The drawing under review shows one solid part. Ordinate dimensions are in mm from its lowest x, y, z. Give positions to 0.01 mm unless a question says otherwise; leave off trailing zeros. Order: outer loops, then holes, each group sorted by start corner. A loop starts at its lowest first (then second) coordinate and runs counter-clockwise, first axis right, second up. Notation, with made-up numbers: (10.5, -38) -> (31.5, -38) arc R29 cw to (31.5, 0) -> close; hole circle Ø1 at (32.5, -3.75). An arc over 180 degrees is marked (long way). Return JSON: item names as keys, results as strings. Group by question number.
1) Add section C-C (y = 0.6). Give the boundary of the cut face in (x, z), then the cut area to 3 significant figures.
2) Add section D-D (x = 48.5). Give the boundary of the cut face in (y, z), then the cut area to 3 significant figures.
3) To check wall thickness, follow line 1 along X through (y, z) = (1.95, 22.75); line 2 along Z through (x, y) = (4, 2); line 3 along X through (y, z) = (2.45, 41.5). State the ranges of each line that lie inside material, in increasing order.
4) Add section B-B (z = 20). Give the boundary of the cut face in (x, y).
5) Add section A-A (x = 4). Give the boundary of the cut face in (y, z).
6) Insertion check: P1, Ø2, axis at x = 4, z = 41.5, coming from the -Y side (3 decimals). The pin has a flat end and moves straight along its axis. Give the tip position at first contact, or say it passes through.
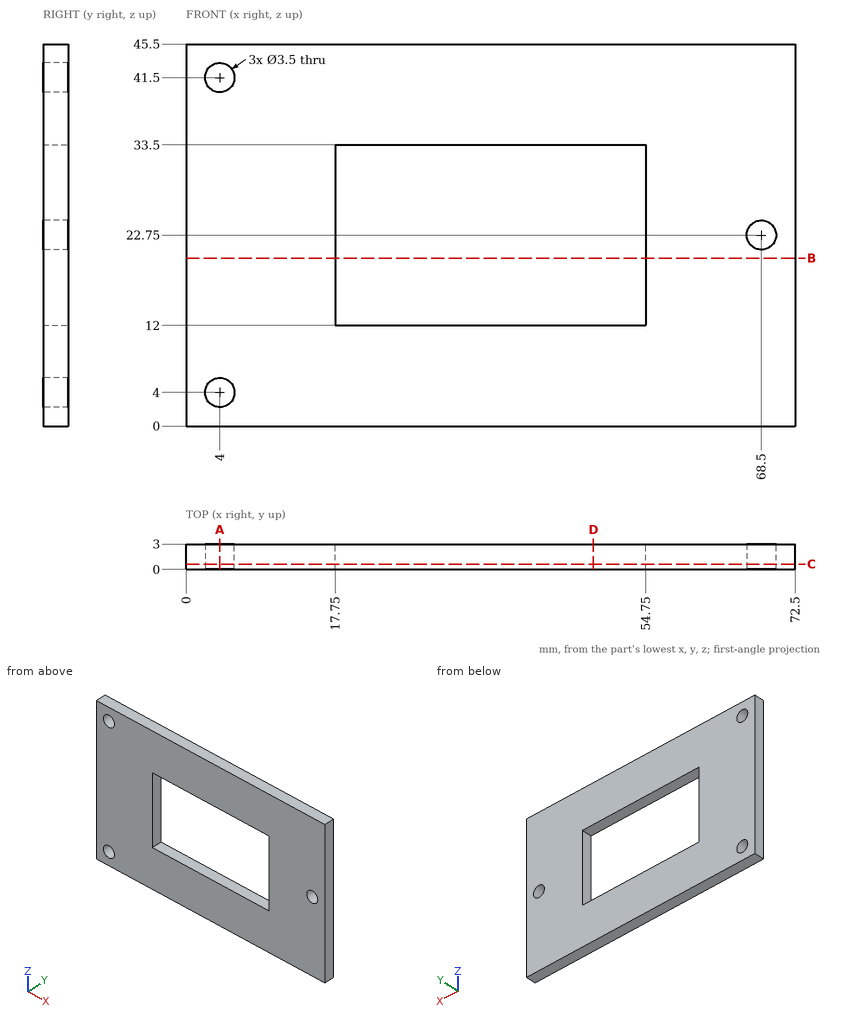
Evaluation:
{
 "1": {"outline": "(0, 0) -> (72.5, 0) -> (72.5, 45.5) -> (0, 45.5) -> close; hole circle Ø3.5 at (4, 4); hole circle Ø3.5 at (4, 41.5); hole (17.75, 12) -> (54.75, 12) -> (54.75, 33.5) -> (17.75, 33.5) -> close; hole circle Ø3.5 at (68.5, 22.75)", "area": "2,470 mm^2"},
 "2": {"outline": "(0, 0) -> (3, 0) -> (3, 12) -> (0, 12) -> close; (0, 33.5) -> (3, 33.5) -> (3, 45.5) -> (0, 45.5) -> close", "area": "72.0 mm^2"},
 "3": {"line 1": "0 to 17.75, 54.75 to 66.75, 70.25 to 72.5", "line 2": "0 to 2.25, 5.75 to 39.75, 43.25 to 45.5", "line 3": "0 to 2.25, 5.75 to 72.5"},
 "4": {"outline": "(0, 0) -> (17.75, 0) -> (17.75, 3) -> (0, 3) -> close; (54.75, 0) -> (72.5, 0) -> (72.5, 3) -> (54.75, 3) -> close"},
 "5": {"outline": "(0, 0) -> (3, 0) -> (3, 2.25) -> (0, 2.25) -> close; (0, 5.75) -> (3, 5.75) -> (3, 39.75) -> (0, 39.75) -> close; (0, 43.25) -> (3, 43.25) -> (3, 45.5) -> (0, 45.5) -> close"},
 "6": {"P1": "through"}
}
